Input: dimensioned drawing with shaded views. Units: mm. Origin: part minimum x, y, z. Round coordinates to 2 decimals unless told otherwise and drop trailing zeros. Loops run counter-clockwise (first coordinate to the right, second up) from the corner with the lowest first, then second, coordinate; pieces in that order, holes last. Notation, with made-up numbers: (16.5, 81) -> (61.5, 81) arc R33 ccw to (61.5, 113) -> close; hole circle Ø7 at (88, -28). An arc over 180 degrees is marked (long way). Answer as a JSON object with one key per item and string values.
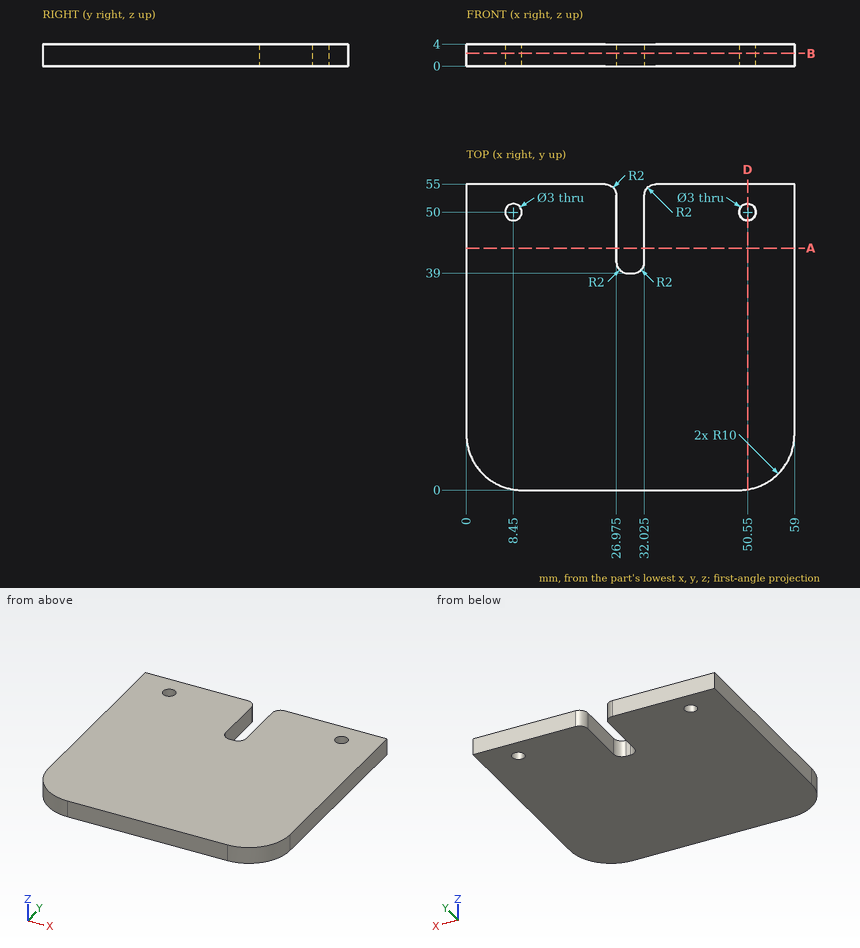
1) Section B-B, the plane z = 2.3. Count the separate pieces of the cut face and the enclosed holes in it, plus the area to 3 significant figures.
Output:
{"separate pieces": "1", "enclosed holes": "2", "area": "3,110 mm^2"}
2) Contact query for flat-ended pins moving along their axis: P1, Ø5, axis at x = 12, y = 26.5, coming from the -Z side; P2, Ø2, axis at x = 50.5, z = 0.5, coming from the -Y side; P3, Ø0.5, axis at x = 29.5, z = 3, coming from the +Y side; P4, Ø2.5, axis at x = 50.55, y = 50, coming from the +Z side. Output: stop coordinate, or through.
Output:
{"P1": "stops at z = 0", "P2": "stops at y = 0.01", "P3": "stops at y = 39", "P4": "passes through"}
3) Ray query, probe 1 along X at (y, z) = (42, 0.4) (1 decimal); probe 2 along Y at (x, z) = (50.55, 2.45); probe 3 along X at (y, z) = (6.5, 3.55). Return the intervals inside material, ascending.
Output:
{"probe 1": "x = 0 to 27, 32 to 59", "probe 2": "y = 0.12 to 48.5, 51.5 to 55", "probe 3": "x = 0.63 to 58.37"}
4) Section D-D, the plane x = 50.55. Output: boundary loops of the cut face in (y, z).
Output:
{"outline": "(0.12, 0) -> (48.5, 0) -> (48.5, 4) -> (0.12, 4) -> close; (51.5, 0) -> (55, 0) -> (55, 4) -> (51.5, 4) -> close"}
5) Section A-A, the plane y = 43.5. Output: boundary loops of the cut face in (x, z) (1 decimal), plus the area to 3 significant figures.
Output:
{"outline": "(0, 0) -> (27, 0) -> (27, 4) -> (0, 4) -> close; (32, 0) -> (59, 0) -> (59, 4) -> (32, 4) -> close", "area": "216 mm^2"}
